For this review, take the finished solid that the model builds, in its own axes (mm). Face numbers are marked on the shaded views. A direction names the side the tool comes from. Give positions to 0.01 mm unless a question says otherwise; leave off trailing zeros. Loops run counter-clockwise (first coordinate to the right, second up) from the corner with the lowest first, then second, coordinate; pieces in that order, holes last. Notation, with made-up numbers: (-22, 54) - (-2, 54) arc R21 cw to (-2, 58) - close; hole circle Ø3 at (46, 17.5). An arc over 180 degrees is marked (long way). Put each result on its own line as item: value.
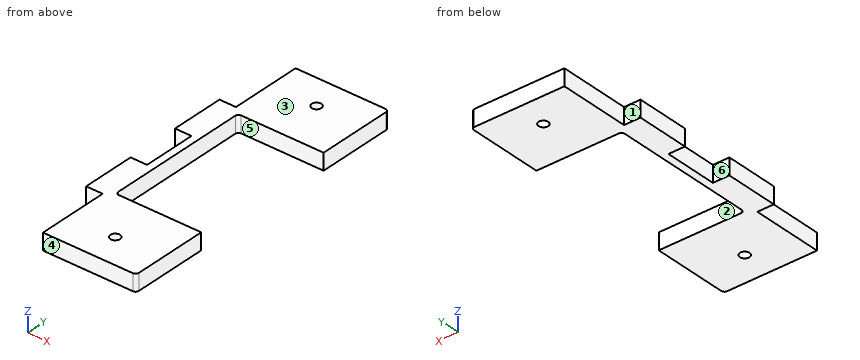
from build123d import *

# Parameters (mm, degrees)
SKETCH1_R           = 1.5
BOSS_EXTRUDE1_DEPTH = 5.13
CUT_EXTRUDE1_REACH  = 7.13


with BuildPart() as part:
    # Sketch1 → Boss-Extrude1 (new body)
    with BuildSketch(Plane.XY):
        with BuildLine():
            Line((-16.470914087, 7.163135174), (-16.470914087, -9.436864826))
            Line((-16.470914087, -9.436864826), (-21.600914087, -9.436864826))
            Line((-21.600914087, -9.436864826), (-21.600914087, -26.036864826))
            Line((-21.600914087, -26.036864826), (-16.470914087, -26.036864826))
            Line((-16.470914087, -26.036864826), (-16.470914087, -48.316864826))
            Line((-16.470914087, -48.316864826), (11.529085913, -48.316864826))
            ThreePointArc((11.529085913, -48.316864826), (12.236192694, -48.023971608), (12.529085913, -47.316864826))
            Line((12.529085913, -47.316864826), (12.529085913, 45.043135174))
            ThreePointArc((12.529085913, 45.043135174), (12.236192694, 45.750241955), (11.529085913, 46.043135174))
            Line((11.529085913, 46.043135174), (-16.470914087, 46.043135174))
            Line((-16.470914087, 46.043135174), (-16.470914087, 23.763135174))
            Line((-16.470914087, 23.763135174), (-21.600914087, 23.763135174))
            Line((-21.600914087, 23.763135174), (-21.600914087, 7.163135174))
            Line((-21.600914087, 7.163135174), (-16.470914087, 7.163135174))
        make_face()
        with Locations((-1.970914087, -38.750864826)):
            Circle(SKETCH1_R, mode=Mode.SUBTRACT)
        with Locations((-1.970914087, 36.477135174)):
            Circle(SKETCH1_R, mode=Mode.SUBTRACT)
    extrude(amount=BOSS_EXTRUDE1_DEPTH)

    # Sketch2 → Cut-Extrude1 (cut, up to next)
    with BuildSketch(Plane.XY.offset(5.13), mode=Mode.PRIVATE) as cut_extrude1_sk1:
        with BuildLine():
            Line((12.529085913, 21.723135174), (-13.140914087, 21.723135174))
            ThreePointArc((-13.140914087, 21.723135174), (-13.848020868, 21.430241955), (-14.140914087, 20.723135174))
            Line((-14.140914087, 20.723135174), (-14.140914087, -22.996864826))
            ThreePointArc((-14.140914087, -22.996864826), (-13.848020868, -23.703971608), (-13.140914087, -23.996864826))
            Line((-13.140914087, -23.996864826), (12.529085913, -23.996864826))
            Line((12.529085913, -23.996864826), (12.529085913, 21.723135174))
        make_face()
    cut_extrude1_tool1 = extrude(cut_extrude1_sk1.sketch, amount=-CUT_EXTRUDE1_REACH, mode=Mode.PRIVATE) & part.part
    add(cut_extrude1_tool1.solids().sort_by_distance((-0.801297, -1.136865, 5.13))[0], mode=Mode.SUBTRACT)


solid = part.part
1) Draft analysis for pull direction Y (two halves, no side actions). For the marked faces 1, 2 and 3, state which applies: pulls with the +Y half, pulls with the -Y half, needs draft (parallel to the pull), parting line crosses it, or undercut.
Geometry check:
face 1: pulls with the +Y half
face 2: undercut
face 3: needs draft
2) Take a section at D-D on y = -21. State the section outline as (x, z) points, and give its area (3 significant figures).
Geometry check:
outline: (-21.6, 0) - (-14.14, 0) - (-14.14, 5.13) - (-21.6, 5.13) - close
area: 38.3 mm²
3) For the marked faces 4, 5 and 6, list the 3-axis set-ups (+Z, -Z, +X, -X, +Y, -Y) from which the entire face can be reached by the end or side of a thin tool; tool diameter is ignored.
Geometry check:
face 4: +Z, -Z, +X, -X, -Y
face 5: +Z, -Z, +X
face 6: +Z, -Z, -X
4) Wall thickness on line 1 (Y direction, x = -18.5, z = 0.85); line 2 (Y direction, x = -11.5, z = 2.85); line 3 (X direction, y = -18, z = 2.8): over which ranges is each line inside the solid? List them lowest first.
Geometry check:
line 1: y = -26.04 to -9.44, 7.16 to 23.76
line 2: y = -48.32 to -24, 21.72 to 46.04
line 3: x = -21.6 to -14.14
5) Take a section at C-C on x = -19. State the section outline as (y, z) points, and give its area (3 significant figures).
Geometry check:
outline: (-26.04, 0) - (-9.44, 0) - (-9.44, 5.13) - (-26.04, 5.13) - close; (7.16, 0) - (23.76, 0) - (23.76, 5.13) - (7.16, 5.13) - close
area: 170 mm²
6) Insertion check: pin 1 Ø2.5 at (x, y) = (-1.97, -38.75) entering from -Z; pin 2 Ø1.5 at (x, z) = (-19.5, 3) entering from +Y; pin 3 Ø2.5 at (y, z) = (32.5, 2) entering from -X; pin 4 Ø12 at (x, y) = (-16.5, -37.5) entering from +Z. Each pin has a flat end and moves straight along its axis. Give the tip position at first contact, or say it passes through.
Geometry check:
pin 1: passes through
pin 2: stops at y = 23.76
pin 3: stops at x = -16.47
pin 4: stops at z = 5.13
7) Take a section at B-B on z = 1.1. State the section outline as (x, y) points, and give its area (3 significant figures).
Geometry check:
outline: (-21.6, -26.04) - (-16.47, -26.04) - (-16.47, -48.32) - (11.53, -48.32) arc R1 ccw to (12.53, -47.32) - (12.53, -24) - (-13.14, -24) arc R1 cw to (-14.14, -23) - (-14.14, 20.72) arc R1 cw to (-13.14, 21.72) - (12.53, 21.72) - (12.53, 45.04) arc R1 ccw to (11.53, 46.04) - (-16.47, 46.04) - (-16.47, 23.76) - (-21.6, 23.76) - (-21.6, 7.16) - (-16.47, 7.16) - (-16.47, -9.44) - (-21.6, -9.44) - close; hole circle Ø3 at (-1.97, -38.75); hole circle Ø3 at (-1.97, 36.48)
area: 1,670 mm²
8) Take a section at A-A on x = 6.5. State the section outline as (y, z) points, and give its area (3 significant figures).
Geometry check:
outline: (-48.32, 0) - (-24, 0) - (-24, 5.13) - (-48.32, 5.13) - close; (21.72, 0) - (46.04, 0) - (46.04, 5.13) - (21.72, 5.13) - close
area: 250 mm²
